Verification items for this drawing (mm, ordinates from the low corner). A direction names the side the tool comes from. Round coordinates to 2 decimals unless told otherwise and drop trailing zeros. Order: outer loops, then holes, each group sorted by start corner. A loop starts at its lowest first (then second) coordinate and runs counter-clockwise, first axis right, second up. Notation, with made-up numbers: (31.5, 74) - (83.5, 74) arc R26 cw to (83.5, 103) - close; hole circle Ø1 at (86.25, -9.75). An arc over 180 degrees is marked (long way). One line per question, with ' | ' between items. Start each with the question number.
Q1. Sectioned sample at D-D, the plane x = 10. Enter the section's corners in (y, z).
Q2. Material ranges on line 1 along Y through (x, z) = (3.5, 7.5); line 2 along Z through (x, y) = (20, 21.9); line 3 along Z through (x, y) = (11.5, 16), recorded low to high.
Q3. Sectioned sample at B-B, the plane y = 12. Enter the section's corners in (x, z).
Q4. Gauge pin test, flat ends, axial feed: P1, Ø5.5, axis at x = 16.5, y = 13, coming from the +Z side; P2, Ø12, axis at y = 21, z = 12.5, coming from the -X side; P3, Ø12, axis at x = 30.5, y = 21, coming from the -Z side; P4, Ø6, axis at y = 20, z = 12, coming from the -X side. Record the tip position at first contact, or that the pin passes through.
Q5. Sectioned sample at A-A, the plane x = 20. Enter the section's corners in (y, z), then the cut area to 3 significant figures.
Q6. Sectioned sample at C-C, the plane z = 30. Enter the section's corners in (x, y).
Q7. Tool access check on the marked faces 4 and 5. Record the directions out of +Z, -Z, +X, -X, +Y, -Y that give a thin tool (end or side, any length) a straight path to the whole face; none if there is none.
Q8. Mould release check, pull along Z, two halves, no side actions. Record for the marked faces 1, 2 and 3: +Z half, -Z half, draft (parallel to the pull), parting line (faces both ways), or undercut.
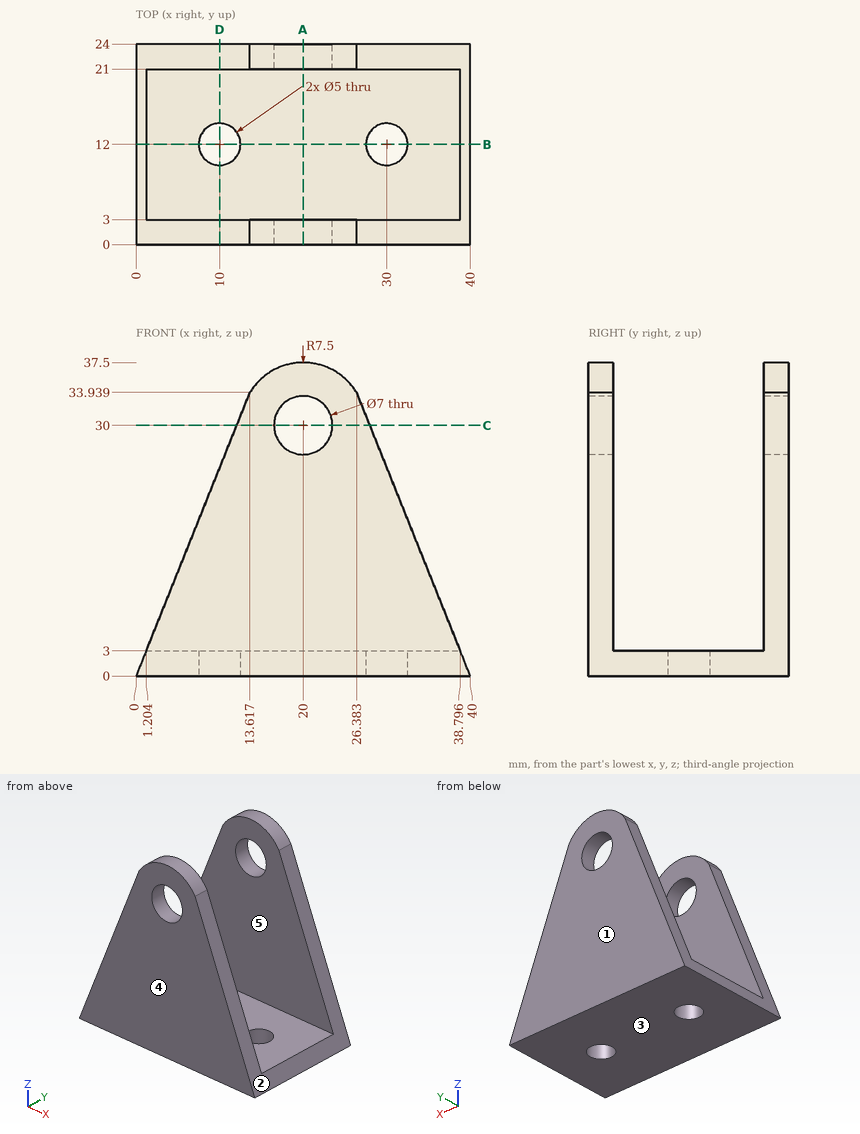
Determined:
1) outline: (0, 0) - (9.5, 0) - (9.5, 3) - (3, 3) - (3, 24.92) - (0, 24.92) - close; (14.5, 0) - (24, 0) - (24, 24.92) - (21, 24.92) - (21, 3) - (14.5, 3) - close
2) line 1: y = 0 to 3, 21 to 24 | line 2: z = 0 to 26.5, 33.5 to 37.5 | line 3: z = 0 to 3
3) outline: (0, 0) - (7.5, 0) - (7.5, 3) - (1.2, 3) - close; (12.5, 0) - (27.5, 0) - (27.5, 3) - (12.5, 3) - close; (32.5, 0) - (40, 0) - (38.8, 3) - (32.5, 3) - close
4) P1: stops at z = 3 | P2: stops at x = 2.61 | P3: stops at z = 0 | P4: stops at x = 3.68
5) outline: (0, 0) - (24, 0) - (24, 26.5) - (21, 26.5) - (21, 3) - (3, 3) - (3, 26.5) - (0, 26.5) - close; (0, 33.5) - (3, 33.5) - (3, 37.5) - (0, 37.5) - close; (21, 33.5) - (24, 33.5) - (24, 37.5) - (21, 37.5) - close | area: 237 mm2
6) outline: (12.04, 0) - (16.5, 0) - (16.5, 3) - (12.04, 3) - close; (12.04, 21) - (16.5, 21) - (16.5, 24) - (12.04, 24) - close; (23.5, 0) - (27.96, 0) - (27.96, 3) - (23.5, 3) - close; (23.5, 21) - (27.96, 21) - (27.96, 24) - (23.5, 24) - close
7) face 4: +Z, -Z, +X, -X, -Y | face 5: +Z, +X, -X
8) face 1: draft | face 2: +Z half | face 3: -Z half
